```python
from build123d import *

# Parameters (mm, degrees)
F0_R      = 31.75
F1_DEPTH  = 114.3
F2_R      = 23.876
F3_DEPTH  = 3.175
F4_R      = 25.4
F5_DEPTH  = 79.375
F6_SIZE   = 1.6002
F7_R      = 50.8
F8_DEPTH  = 44.45
F9_SIZE   = 12.7
F10_R     = 31.75
F11_DEPTH = 768.35
F12_R     = 26.9875
F13_DEPTH = 114.3
F14_R     = 23.876
F15_DEPTH = 3.175
F16_R     = 25.4
F17_DEPTH = 79.375
F18_SIZE  = 1.6002


with BuildPart() as f1:
    # F0 (on Top) → F1 (new body)
    with BuildSketch(Plane.XY):
        Circle(F0_R)
    extrude(amount=-F1_DEPTH)

    # F2 (on face) → F3 (join)
    with BuildSketch(Plane(origin=(0, 0, -114.3), x_dir=(1, 0, 0), z_dir=(0, 0, -1))):
        Circle(F2_R)
    extrude(amount=F3_DEPTH)

    # F4 (on face) → F5 (join)
    with BuildSketch(Plane(origin=(0, 0, -117.475), x_dir=(1, 0, 0), z_dir=(0, 0, -1))):
        Circle(F4_R)
    extrude(amount=F5_DEPTH)

    # F6
    f6_edges = [f1.edges().sort_by_distance(p)[0] for p in [
        (-25.4, 0, -196.85),
    ]]
    chamfer(f6_edges, length=F6_SIZE)

    # F7 (on face) → F8 (join)
    with BuildSketch(Plane.XY):
        Circle(F7_R)
    extrude(amount=F8_DEPTH)

    # F9
    f9_edges = [f1.edges().sort_by_distance(p)[0] for p in [
        (-50.8, 0, 44.45),
    ]]
    chamfer(f9_edges, length=F9_SIZE)

    # F10 (on face) → F11 (join)
    with BuildSketch(Plane.XY.offset(44.45)):
        Circle(F10_R)
    extrude(amount=F11_DEPTH)

    # F12 (on face) → F13 (join)
    with BuildSketch(Plane.XY.offset(812.8)):
        Circle(F12_R)
    extrude(amount=F13_DEPTH)

    # F14 (on face) → F15 (join)
    with BuildSketch(Plane.XY.offset(927.1)):
        Circle(F14_R)
    extrude(amount=F15_DEPTH)

    # F16 (on face) → F17 (join)
    with BuildSketch(Plane.XY.offset(930.275)):
        Circle(F16_R)
    extrude(amount=F17_DEPTH)

    # F18
    f18_edges = [f1.edges().sort_by_distance(p)[0] for p in [
        (-25.4, 0, 1009.65),
    ]]
    chamfer(f18_edges, length=F18_SIZE)


solid = f1.part
```
Input: part model. Units: mm. Frame: model coordinates. A direction names the side the tool comes from. Coordinates: 2 decimals unless noted, no trailing zeros. Write each loop counter-clockwise with the first axis right and the second up, starting at its lowest first coordinate (ties: lowest second). Pieces come first, ordered by that corner, then holes. Notation, with made-up numbers: (35, 18) -> (91, 18) arc R23 cw to (91, 36) -> close; hole circle Ø9 at (89, 33.25). An arc over 180 degrees is marked (long way). Write each question's results on one line, items separated by ' | '.
Item 1: Section query A-A on z = 684. Return loops of the section in (x, y), plus the area to 3 significant figures.
Conclusion:
outline: circle Ø63.5 at (0, 0) | area: 3,170 mm^2
Item 2: Set-up query: faces 1 (the cylindrical face through (-6.883, -30.995, 423.247)), 2 (the flat face through (21.9, 23.3, 0)), 3 (the flat face through (19, -15, 930.275)). Return all of +Z, -Z, +X, -X, +Y, -Y with unobstructed straight access to the full face (end or side cutting, diameter ignored); none if empty.
Conclusion:
face 1: +Z | face 2: -Z | face 3: none
Item 3: Pin query (flat end, axial travel): pin 1 Ø1 at (y, z) = (-12.5, 200) entering from +X; pin 2 Ø1 at (x, y) = (21.5, 35) entering from -Z; pin 3 Ø10 at (y, z) = (33, 76.5) entering from +X. Return the tip coordinate at first contact, or that it passes through.
Conclusion:
pin 1: stops at x = 29.39 | pin 2: stops at z = 0 | pin 3: stops at x = 14.97
Item 4: Material intervals for probe 1 along Z at (x, y) = (-28, 24); probe 2 along X at (y, z) = (-3, 703); probe 3 along X at (y, z) = (-21, 813), sorted ascending.
Conclusion:
probe 1: z = 0 to 44.45 | probe 2: x = -31.61 to 31.61 | probe 3: x = -16.95 to 16.95
Item 5: Mould query, pull axis Z, two halves, no side actions, for faces 4 (the cylindrical face through (-19.89, 18.24, 869.15)), 5 (the flat face through (0, 0, 1009.65)), 6 (the cylindrical face through (-5.176, 23.308, -115.865)). Classes: +Z half, -Z half, draft (parallel to the pull), parting line (faces both ways), or undercut.
Conclusion:
face 4: draft | face 5: +Z half | face 6: undercut
